The drawing under review shows one solid part. Ordinate dimensions are in mm from its lowest x, y, z. A direction names the side the tool comes from. Coordinates: 2 decimals unless noted, no trailing zeros. Loops run counter-clockwise (first coordinate to the right, second up) from the corner with the lowest first, then second, coordinate; pieces in that order, holes last. Notation, with made-up numbers: (-5.5, -9.5) - (36.5, -9.5) arc R35 cw to (36.5, 22.5) - close; hole circle Ø2 at (20.25, 83). An arc over 180 degrees is marked (long way). Use one line per item in the form item = value. Start each with the question number.
1. For pin 1 Ø12.5 at (x, z) = (64, 8) entering from -Y; pin 2 Ø5 at (y, z) = (81, 20.5) entering from -X, all flat-tipped, find the tip position at first contact; note any pin that passes through.
2. Add section B-B on x = 100. Give the boundary of the cut face in (y, z).
3. Add section D-D on x = 30. Give the boundary of the cut face in (y, z), and give its area (4 significant figures).
4. Add section A-A on z = 23.25. Give the boundary of the cut face in (x, y).
5. Draft analysis for pull direction X (two halves, no side actions). For the marked faces 1, 2 and 3, state which applies: +X half, -X half, draft (parallel to the pull), parting line (faces both ways), or undercut.
6. Machinability: for the marked faces 4, 5 and 6, which of the approach directions +Z, -Z, +X, -X, +Y, -Y give a long, thin tool a straight path to every point of the face, cutting with its end or side? Answer none if there is none.
7. To check wall thickness, follow probe 1 along Y at (x, z) = (100, 13); probe 2 along X at (y, z) = (83.5, 21.75); probe 3 along X at (y, z) = (41, 2.25). State the ranges of each line that lie inside material, in increasing order.
8. Add section C-C on y = 24.5. Give the boundary of the cut face in (x, z), and give its area (3 significant figures).
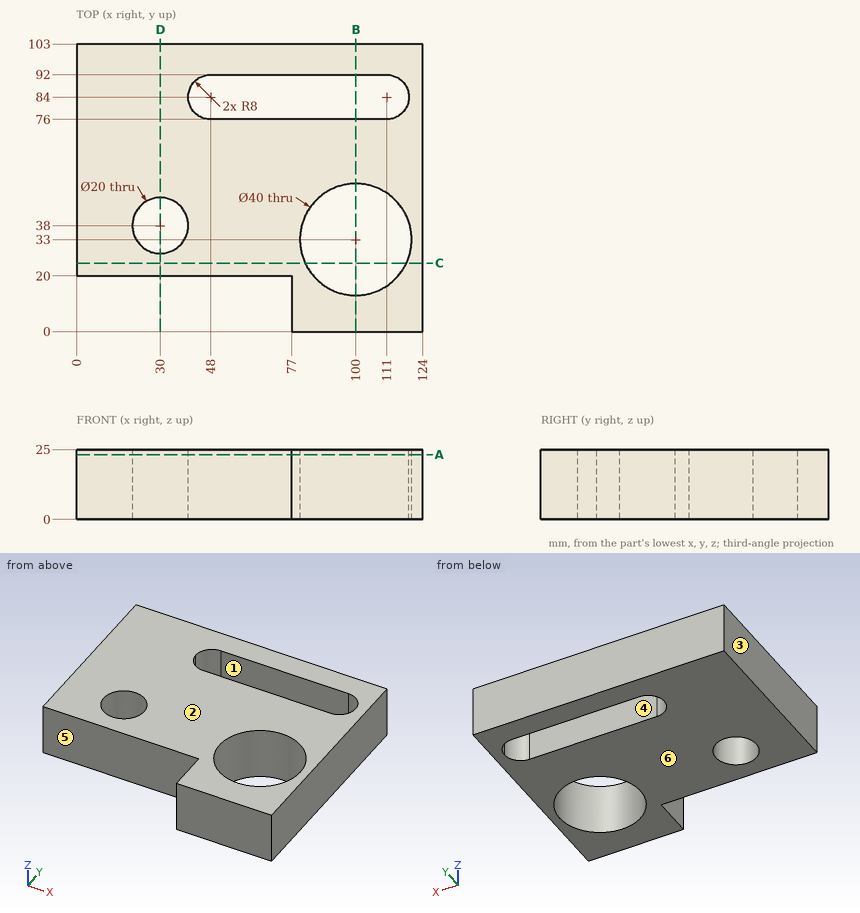
Conclusion:
q1.pin_1 = 20
q1.pin_2 = 0
q2.outline = (0, 0) - (13, 0) - (13, 25) - (0, 25) - close; (53, 0) - (76, 0) - (76, 25) - (53, 25) - close; (92, 0) - (103, 0) - (103, 25) - (92, 25) - close
q3.outline = (20, 0) - (28, 0) - (28, 25) - (20, 25) - close; (48, 0) - (103, 0) - (103, 25) - (48, 25) - close
q3.area = 1,575 mm^2
q4.outline = (0, 20) - (77, 20) - (77, 0) - (124, 0) - (124, 103) - (0, 103) - close; hole circle Ø20 at (30, 38); hole (40, 84) arc R8 ccw to (48, 76) - (111, 76) arc R8 ccw to (119, 84) arc R8 ccw to (111, 92) - (48, 92) arc R8 ccw to start; hole circle Ø40 at (100, 33)
q5.face_1 = undercut
q5.face_2 = draft
q5.face_3 = -X half
q6.face_4 = +Z, -Z
q6.face_5 = +Z, -Z, -X, -Y
q6.face_6 = -Z, +X, -X, +Y, -Y
q7.probe_1 = 0 to 13, 53 to 76, 92 to 103
q7.probe_2 = 0 to 40.02, 118.98 to 124
q7.probe_3 = 0 to 20.46, 39.54 to 81.67, 118.33 to 124
q8.outline = (0, 0) - (81.9, 0) - (81.9, 25) - (0, 25) - close; (118.1, 0) - (124, 0) - (124, 25) - (118.1, 25) - close
q8.area = 2,190 mm^2
